Job drawing, mm, ordinate dimensions from the low corner. One solid piece. Round coordinates to 2 decimals unless told otherwise and drop trailing zeros. Loops run counter-clockwise (first coordinate to the right, second up) from the corner with the lowest first, then second, coordinate; pieces in that order, holes last.
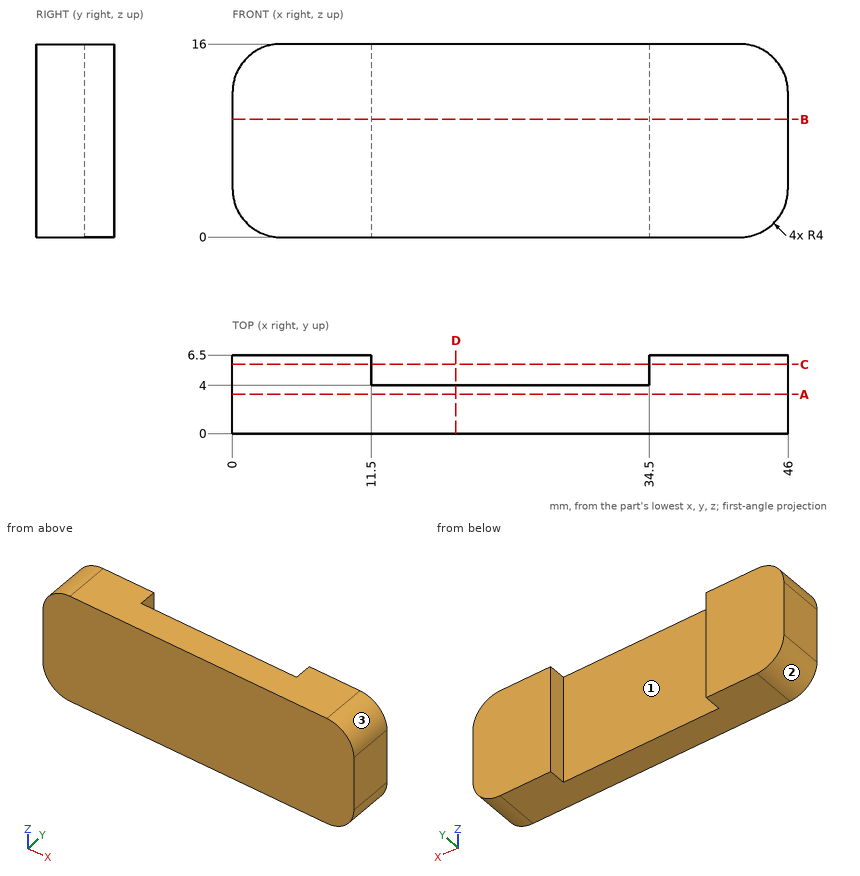
1) Slice it at B-B, the plane z = 9.75. Give the cut face in (x, y), then the cut area to 4 significant figures.
Values:
outline: (0, 0) - (46, 0) - (46, 6.5) - (34.5, 6.5) - (34.5, 4) - (11.5, 4) - (11.5, 6.5) - (0, 6.5) - close
area: 241.5 mm2
2) Slice it at A-A, the plane y = 3.25. Give the cut face in (x, z).
Values:
outline: (0, 4) arc R4 ccw to (4, 0) - (42, 0) arc R4 ccw to (46, 4) - (46, 12) arc R4 ccw to (42, 16) - (4, 16) arc R4 ccw to (0, 12) - close
3) Drop a flat-ended pin along its axis: pin 1 Ø8 at (x, z) = (18.5, 11) entering from +Y. Give the stop position or say it passes through.
Values:
pin 1: stops at y = 4
4) Slice it at C-C, the plane y = 5.75. Give the cut face in (x, z), then the cut area to 3 significant figures.
Values:
outline: (0, 4) arc R4 ccw to (4, 0) - (11.5, 0) - (11.5, 16) - (4, 16) arc R4 ccw to (0, 12) - close; (34.5, 0) - (42, 0) arc R4 ccw to (46, 4) - (46, 12) arc R4 ccw to (42, 16) - (34.5, 16) - close
area: 354 mm2
5) Mould opens along X. For the marked faces 1, 2 and 3 say: released by +X, released by -X, zero draft, split by the parting line, or undercut.
Values:
face 1: undercut
face 2: released by -X
face 3: released by +X
6) Slice it at D-D, the plane x = 18.5. Give the cut face in (y, z), then the cut area to 3 significant figures.
Values:
outline: (0, 0) - (4, 0) - (4, 16) - (0, 16) - close
area: 64.0 mm2
7) Wall check: line 1 along X through (y, z) = (4.75, 10); line 2 along Y through (x, z) = (16.5, 3.25); line 3 along X through (y, z) = (5.5, 15). Give the ranges that are in metal, low to high.
Values:
line 1: x = 0 to 11.5, 34.5 to 46
line 2: y = 0 to 4
line 3: x = 1.35 to 11.5, 34.5 to 44.65
